Can you work these out from the model? Positions are in its coordinate system, mm. A direction names the side the tool comes from. Round coordinates to 2 decimals unless told otherwise and drop trailing zeros. Loops run counter-clockwise (first coordinate to the right, second up) from the corner with the lowest first, then second, coordinate; pieces in that order, holes last. Notation, with made-up numbers: M 40.25,25 L 86.25,25 A16 cw 86.25,45 Z; hole C -30.5,70 d9. An arc over 180 degrees is marked long. Return JSON: item names as keys, results as strings.
```python
from build123d import *

# Parameters (mm, degrees)
EXTRUDE_2_DEPTH     = 2
SKETCH_2_R          = 32
EXTRUDE_3_DEPTH     = 18
SKETCH_10_W         = 1.025
SKETCH_10_H         = 37.5
HOLE_WIZARD_M4_2_D  = 3.3
HOLE_WIZARD_M60_2_D = 58.5


with BuildPart() as part:
    # 草图1 → 凸台-拉伸2 (new body)
    with BuildSketch(Plane(origin=(0, 0, 0), x_dir=(1, 0, 0), z_dir=(0, 1, 0))):
        with BuildLine():
            ThreePointArc((36.247895087, 36.674436315), (42.841106398, 35.700921998), (42.609721719, 29.040244357))
            ThreePointArc((42.609721719, 29.040244357), (34.804095286, 18.178082868), (34.668896044, 4.802879043))
            ThreePointArc((34.668896044, 4.802879043), (35, 0), (34.668896044, -4.802879043))
            ThreePointArc((34.668896044, -4.802879043), (34.804095286, -18.178082868), (42.609721719, -29.040244357))
            ThreePointArc((42.609721719, -29.040244357), (42.841106398, -35.700921998), (36.247895087, -36.674436315))
            ThreePointArc((36.247895087, -36.674436315), (24.15622984, -30.955521404), (10.97591146, -33.234460544))
            ThreePointArc((10.97591146, -33.234460544), (0, -35), (-10.97591146, -33.234460544))
            ThreePointArc((-10.97591146, -33.234460544), (-24.15622984, -30.955521404), (-36.247895087, -36.674436315))
            ThreePointArc((-36.247895087, -36.674436315), (-42.841106398, -35.700921998), (-42.609721719, -29.040244357))
            ThreePointArc((-42.609721719, -29.040244357), (-34.804095286, -18.178082868), (-34.668896044, -4.802879043))
            ThreePointArc((-34.668896044, -4.802879043), (-35, 0), (-34.668896044, 4.802879043))
            ThreePointArc((-34.668896044, 4.802879043), (-34.804095286, 18.178082868), (-42.609721719, 29.040244357))
            ThreePointArc((-42.609721719, 29.040244357), (-42.841106398, 35.700921998), (-36.247895087, 36.674436315))
            ThreePointArc((-36.247895087, 36.674436315), (-24.15622984, 30.955521404), (-10.97591146, 33.234460544))
            ThreePointArc((-10.97591146, 33.234460544), (0, 35), (10.97591146, 33.234460544))
            ThreePointArc((10.97591146, 33.234460544), (24.15622984, 30.955521404), (36.247895087, 36.674436315))
        make_face()
    extrude(amount=EXTRUDE_2_DEPTH)

    # 草图2 → 凸台-拉伸3 (add)
    with BuildSketch(Plane(origin=(0, 2, 0), x_dir=(1, 0, 0), z_dir=(0, 1, 0))):
        with Locations(Location((0, 0, 0), (0, 0, 270))):
            Circle(SKETCH_2_R)
    extrude(amount=EXTRUDE_3_DEPTH)

    # 草图10 → M2.5 螺纹孔1 (revolve, cut)
    with BuildSketch(Plane(origin=(0, 16, 0), x_dir=(0, 1, 0), z_dir=(1, 0, 0))):
        with Locations((0.5125, 18.75)):
            Rectangle(SKETCH_10_W, SKETCH_10_H)
    hole_wizard_m2_5_1 = revolve(axis=Axis((0, 16, -6.35), (0, 0, 1)), mode=Mode.SUBTRACT)

    # 镜向3: M2.5 螺纹孔1 across plane
    add(hole_wizard_m2_5_1.mirror(Plane.XY), mode=Mode.SUBTRACT)

    # M4 螺纹孔2 (through all)
    with Locations(Plane(origin=(0, 20, 0), x_dir=(1, 0, 0), z_dir=(0, 1, 0))):
        with Locations((-39, 32.5), (-39, -32.5), (39, -32.5), (39, 32.5)):
            Hole(HOLE_WIZARD_M4_2_D / 2)

    # M60 螺纹孔2 (through all)
    with Locations(Plane(origin=(0, 20, 0), x_dir=(1, 0, 0), z_dir=(0, 1, 0))):
        with Locations((0, 0)):
            Hole(HOLE_WIZARD_M60_2_D / 2)


solid = part.part
```
Q1. On a 3-axis mill with a long thin cutter (end or side, diameter ignored), from which of +Z, -Z, +X, -X, +Y, -Y can I reach the whole of each face in a straight line? I mean faces 1 (the cylindrical face through (-38.785, 0.986, 30.864)), 2 (the flat face through (26, 2, 19)). Say none if no direction works.
Results:
{"face 1": "+Y, -Y", "face 2": "+Y"}
Q2. If I drill on line 1 along X through (y, z) = (1.2, 32.5); line 2 along Z through (x, y) = (-39, 0.6); line 3 along X through (y, z) = (15.5, -23.5), over which ranges is the centre line in solid material (lowest first)?
Results:
{"line 1": "x = -44 to -40.65, -37.35 to -29.79, -12.54 to 12.54, 29.79 to 37.35, 40.65 to 44", "line 2": "z = -37.5 to -34.15, -30.85 to -25.66, 25.66 to 30.85, 34.15 to 37.5", "line 3": "x = -21.72 to -17.42, 17.42 to 21.72"}
Q3. Suppose I cut it at A-A, the plane x = 0. Please give me the cut outline in (y, z) (3 decimals), plus the area to 3 significant figures.
Results:
{"outline": "M 0,-35 L 2,-35 L 2,-32 L 14.975,-32 L 14.975,-29.25 L 0,-29.25 Z; M 0,29.25 L 14.975,29.25 L 14.975,32 L 2,32 L 2,35 L 0,35 Z; M 17.025,-32 L 20,-32 L 20,-29.25 L 17.025,-29.25 Z; M 17.025,29.25 L 20,29.25 L 20,32 L 17.025,32 Z", "area": "111 mm2"}
Q4. I'm going to push flat-ended pins straight in: pin 1 Ø3 at (x, z) = (-39, 32.5) entering from +Y; pin 2 Ø1 at (x, y) = (30, 3.5) entering from +Z; pin 3 Ø3.5 at (x, y) = (0, 16) entering from -Z; pin 4 Ø5 at (x, y) = (2, 17) entering from +Z. Where does each tip first touch, or does it pass through?
Results:
{"pin 1": "passes through", "pin 2": "stops at z = 12.4", "pin 3": "stops at z = -32", "pin 4": "stops at z = 32"}
Q5. Suppose I cut it at D-D, the plane y = 10.75. Please give me the cut outline in (x, z).
Results:
{"outline": "C 0,0 d64; hole C 0,0 d58.5"}
Q6. Suppose I cut it at B-B, the plane z = 14.5. Please give me the cut outline in (x, y).
Results:
{"outline": "M -33.94,0 L -25.4,0 L -25.4,20 L -28.53,20 L -28.53,2 L -33.94,2 Z; M 25.4,0 L 33.94,0 L 33.94,2 L 28.53,2 L 28.53,20 L 25.4,20 Z"}
Q7. Suppose I cut it at C-C, the plane x = -19. Please give me the cut outline in (y, z).
Results:
{"outline": "M 0,-30.86 L 2,-30.86 L 2,-25.75 L 20,-25.75 L 20,-22.24 L 0,-22.24 Z; M 0,22.24 L 20,22.24 L 20,25.75 L 2,25.75 L 2,30.86 L 0,30.86 Z"}
Q8. Thinking about a two-plate mould opening in Z: for faces 3 (the cylindrical face through (42.775, 0.986, -35.779)), 4 (the cylindrical face through (-42.906, 0.986, -35.622)), 5 (the cylindrical face through (-23.97, 0.99, 30.93)), 6 (the cylindrical face through (23.97, 0.99, -30.93)), which applies, pulls with the +Z half, pulls with the -Z half, needs draft (parallel to the pull), parting line crosses it, or undercut?
Results:
{"face 3": "undercut", "face 4": "undercut", "face 5": "pulls with the +Z half", "face 6": "pulls with the -Z half"}
